Verification items for the finished model (mm, model axes). Round coordinates to 2 decimals unless told otherwise and drop trailing zeros. Write each loop counter-clockwise with the first axis right and the second up, starting at its lowest first coordinate (ties: lowest second). Pieces come first, ordered by that corner, then holes. Notation, with made-up numbers: (-1.5, 10) - (34.5, 10) arc R15 ccw to (34.5, 37) - close; hole circle Ø3 at (-6.5, 2). An arc over 180 degrees is marked (long way). Write each question's results on one line, items separated by ' | '.
```python
from build123d import *

# Parameters (mm, degrees)
F2_R    = 5
F3_SIZE = 1


with BuildPart() as f1:
    # F0 (on Right) → F1 (revolve)
    with BuildSketch(Plane.YZ):
        with BuildLine():
            Line((0, 12.5), (0, 0))
            Line((0, 0), (185, 0))
            Line((185, 0), (185, 39))
            Line((185, 39), (1365, 39))
            Line((1365, 39), (1365, 0))
            Line((1365, 0), (1550, 0))
            Line((1550, 0), (1550, 12.5))
            Line((1550, 12.5), (1450, 12.5))
            Line((1450, 12.5), (1450, 45))
            Line((1450, 45), (1415, 45))
            Line((1415, 45), (1389.02606, 35.546259))
            ThreePointArc((1389.02606, 35.546259), (1386.279271, 35.907881), (1385, 38.365337))
            Line((1385, 38.365337), (1385, 45))
            Line((1385, 45), (165, 45))
            Line((165, 45), (165, 38.365337))
            ThreePointArc((165, 38.365337), (163.720729, 35.907881), (160.97394, 35.546259))
            Line((160.97394, 35.546259), (135, 45))
            Line((135, 45), (100, 45))
            Line((100, 45), (100, 12.5))
            Line((100, 12.5), (0, 12.5))
        make_face()
    revolve(axis=Axis((0, 1457.5, 0), (0, -1, 0)))

    # F2
    f2_edges = [f1.edges().sort_by_distance(p)[0] for p in [
        (0, 1450, -12.5),
        (0, 100, -12.5),
    ]]
    fillet(f2_edges, radius=F2_R)

    # F3
    f3_edges = [f1.edges().sort_by_distance(p)[0] for p in [
        (0, 1450, -45),
        (0, 1550, -12.5),
        (0, 0, -12.5),
        (0, 100, -45),
    ]]
    chamfer(f3_edges, length=F3_SIZE)


solid = f1.part
```
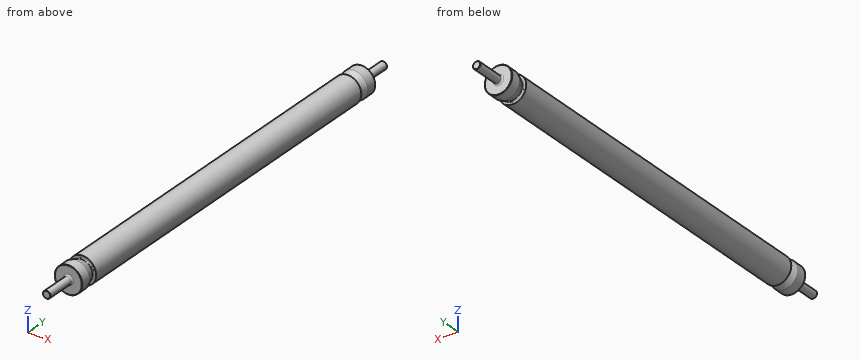
(1) Thickness scan on L1, parallel to Y at x = -33, z = 4.5; L2, parallel to X at y = 1110, z = 2; L3, parallel to Z at x = 0, y = 465.5. Record the ranges inside material, lowest first.
Answer:
L1: 100 to 185, 1365 to 1450 | L2: -44.96 to -38.95, 38.95 to 44.96 | L3: -45 to -39, 39 to 45
(2) Section check A-A (y = 519.5). Record the cut outline in (x, z), plus the area to 3 significant figures.
Answer:
outline: circle Ø90 at (0, 0); hole circle Ø78 at (0, 0) | area: 1,580 mm2
(3) Go/stop test with flat-tipped pins: pin 1 Ø1.5 at (x, y) = (23.5, 715) entering from +Z; pin 2 Ø8 at (x, z) = (1, -18) entering from -Y; pin 3 Ø4 at (x, z) = (-11.5, 11.5) entering from +Y; pin 4 Ø4 at (x, y) = (2, 231.5) entering from -Z. Record where each tip stops, or that it passes through.
Answer:
pin 1: z = 38.83 | pin 2: y = 98.6 | pin 3: y = 1451.19 | pin 4: z = -45
